Check sheet for the modelled part. Datum: model origin and axes. Units: mm. A direction names the side the tool comes from. Coordinates: 2 decimals unless noted, no trailing zeros. Write each loop counter-clockwise with the first axis right and the second up, starting at its lowest first coordinate (ties: lowest second). Pieces come first, ordered by that corner, then holes. Notation, with made-up numbers: (28.5, 19.25) - (54.5, 19.25) arc R16 cw to (54.5, 49.25) - close; hole circle Ø10 at (27, -19.5). An arc over 180 degrees is marked (long way). Use one line per item in the form item = value. Start each with the question number.
1. Scan lines: line 1 along Z through (x, y) = (-11, 14); line 2 along Z through (x, y) = (0, 13.5); line 3 along X through (y, z) = (8.5, -9.75). Record each from-to range of solid material in increasing order.
2. Cross-section at C-C on z = 0. Record the boundary of the cut face in (x, y), then the cut area to 3 significant figures.
3. Cross-section at A-A on x = -13.5. Record the boundary of the cut face in (y, z), then the cut area to 3 significant figures.
4. Cross-section at B-B on y = 10. Give the number of separate pieces and of enclosed holes in the cut face, then the cut area to 3 significant figures.
5. Tool access check on faces 4 (the face through (2, 9.61, -10.92)), 5 (the face through (-16.14, 7.693, -8.768)), 6 (the face through (-14, 7, 10)), 7 (the face through (-14, 7, -7.5)). Record the directions out of +Z, -Z, +X, -X, +Y, -Y that give a thin tool (end or side, any length) a straight path to the whole face; none if there is none.
6. Draft check along Y on faces 1 (the face through (-16, 7, -10)), 2 (the face through (-3.79, 20, -11.14)), 3 (the face through (-16.14, 7.693, 8.733)). Enter one of: +Y half, -Y half, draft (parallel to the pull), parting line (faces both ways), or undercut.
7. Go/stop test with flat-tipped pins: pin 1 Ø1 at (y, z) = (16.5, 4) entering from -X; pin 2 Ø5.5 at (x, y) = (-12.5, 5) entering from +Z; pin 3 Ø3.5 at (x, y) = (-13, 5.5) entering from -Z. Record where each tip stops, or that it passes through.
```python
from build123d import *

# Parameters (mm, degrees)
BOSS_EXTRU_1_DEPTH      = 20
ESQUISSE2_R             = 2.6
ENL_V_MAT_EXTRU_1_DEPTH = 38.127165776
CONG_2_R                = 0.5


with BuildPart() as part:
    # Esquisse1 → Boss.-Extru.1 (new body)
    with BuildSketch(Plane(origin=(0, 0, 0), x_dir=(1, 0, 0), z_dir=(0, 1, 0))):
        with BuildLine():
            Line((-8.182909018, 7.5), (-19.940321926, 7.5))
            Line((-19.940321926, 7.5), (-19.940321926, 10))
            Line((-19.940321926, 10), (-9.940321926, 10))
            ThreePointArc((-9.940321926, 10), (2.269289353, 13.916189343), (12.602252252, 6.324020728))
            ThreePointArc((12.602252252, 6.324020728), (17.6, 0), (12.602252252, -6.324020728))
            ThreePointArc((12.602252252, -6.324020728), (2.269289353, -13.916189343), (-9.940321926, -10))
            Line((-9.940321926, -10), (-19.940321926, -10))
            Line((-19.940321926, -10), (-19.940321926, -7.5))
            Line((-19.940321926, -7.5), (-8.182909018, -7.5))
            ThreePointArc((-8.182909018, -7.5), (1.843161538, -10.945901313), (10.187837838, -4.406581463))
            ThreePointArc((10.187837838, -4.406581463), (15.6, 0), (10.187837838, 4.406581463))
            ThreePointArc((10.187837838, 4.406581463), (1.843161538, 10.945901313), (-8.182909018, 7.5))
        make_face()
    extrude(amount=BOSS_EXTRU_1_DEPTH)

    # Esquisse2 → Enlèv. mat.-Extru.1 (cut, through all)
    with BuildSketch(Plane(origin=(0, 0, -10), x_dir=(-1, 0, 0), z_dir=(0, 0, -1))):
        with Locations((14.940321926, 10)):
            Circle(ESQUISSE2_R)
    extrude(amount=-ENL_V_MAT_EXTRU_1_DEPTH, mode=Mode.SUBTRACT)

    # Congé2
    cong_2_edges = [part.edges().sort_by_distance(p)[0] for p in [
        (-19.940321926, 20, -8.75),
        (-14.061615472, 20, -7.5),
        (12.602252252, 10, -6.324020728),
        (12.602252252, 10, 6.324020728),
        (-9.940321926, 10, 10),
        (1.843161538, 20, -10.945901313),
        (-19.940321926, 10, 10),
        (-19.940321926, 10, 7.5),
        (-19.940321926, 10, -7.5),
        (-19.940321926, 10, -10),
        (15.6, 20, 0),
        (1.843161538, 20, 10.945901313),
        (-14.061615472, 20, 7.5),
        (-19.940321926, 20, 8.75),
        (-14.940321926, 20, 10),
        (2.269289353, 20, 13.916189343),
        (17.6, 20, 0),
        (2.269289353, 20, -13.916189343),
        (-14.940321926, 20, -10),
    ]]
    fillet(cong_2_edges, radius=CONG_2_R)


solid = part.part
```
Final values:
q1.line_1 = -10 to -7.5, 7.5 to 10
q1.line_2 = -14.1 to -11.1, 11.1 to 14.1
q1.line_3 = -19.87 to -17.06, -12.82 to -5.31, 5.31 to 10.19
q2.outline = (15.6, 0) - (17.6, 0) - (17.6, 19.5) arc R0.5 ccw to (17.1, 20) - (16.1, 20) arc R0.5 ccw to (15.6, 19.5) - close
q2.area = 39.9 mm²
q3.outline = (0, -10) - (7.84, -10) - (7.84, -7.5) - (0, -7.5) - close; (0, 7.5) - (7.84, 7.5) - (7.84, 10) - (0, 10) - close; (12.16, -10) - (19.5, -10) arc R0.5 ccw to (20, -9.5) - (20, -8) arc R0.5 ccw to (19.5, -7.5) - (12.16, -7.5) - close; (12.16, 7.5) - (19.5, 7.5) arc R0.5 ccw to (20, 8) - (20, 9.5) arc R0.5 ccw to (19.5, 10) - (12.16, 10) - close
q3.area = 78.1 mm²
q4.separate_pieces = 3
q4.enclosed_holes = 0
q4.area = 207 mm²
q5.face_4 = +Y, -Y
q5.face_5 = +Z, -Z
q5.face_6 = +Z, -X, +Y, -Y
q5.face_7 = -X, +Y, -Y
q6.face_1 = draft
q6.face_2 = +Y half
q6.face_3 = undercut
q7.pin_1 = 10.15
q7.pin_2 = 10.19
q7.pin_3 = -10
